Source: CAD feature listing. Evaluate the final solid. Frame: model axes, mm. A direction names the side the tool comes from. Round coordinates to 2 decimals unless told otherwise and drop trailing zeros. Order: outer loops, then holes, each group sorted by start corner. A loop starts at its lowest first (then second) coordinate and runs counter-clockwise, first axis right, second up. Notation, with made-up numbers: M 45,45 L 66,45 A4 cw 66,52 Z; hole C 76,72.5 d3. An arc over 180 degrees is marked long. Answer as CSV lines item,"result". Start each with the question number.
Item 1: Section query A-A on z = 0. Return the cut outline in (x, y), plus the area to 3 significant figures.
Item 2: First-contact query: P1, Ø8, axis at x = 7.5, z = -4, coming from the -Y side; P2, Ø2.5, axis at x = 6.36, z = -6.36, coming from the -Y side; P3, Ø10, axis at y = 29.5, z = -3, coming from the -X side. Flat tips, straight axial feed; report the tip coordinate or a pass-through.
Item 3: Section query C-C on z = -9.5. Return the cut outline in (x, y).
Item 4: Line query: line 1 (Y direction, x = 5.25, z = -6.5); line 2 (Z direction, x = 2, y = 15); line 3 (Y direction, x = 6, z = -6.5). Output: solid intervals per line, ascending. Write a range as [from, to].
Item 5: Section query D-D on z = -4.25. Return the cut outline in (x, y).
Item 6: Section query B-B on y = 23. Return the cut outline in (x, z).
Item 7: Set-up query: faces 4 (the face through (-6, -1, 0)), 5 (the face through (0, -1, -7)), 6 (the face through (5.57, 1.48, -6.97)), 7 (the face through (2.341, 39.544, -10.543)). Return all of +Z, -Z, +X, -X, +Y, -Y with unobstructed straight access to the full face (end or side cutting, diameter ignored); none if empty.
Item 8: Pull-direction query (X, two-part tool) for faces 1 (the face through (-6, 3, -6)), 2 (the face through (0, -1, 7)), 3 (the face through (6, -1, 0)); classes: +X half, -X half, draft (parallel to the pull), parting line (faces both ways), or undercut.
from build123d import *

# Parameters (mm, degrees)
F0_R      = 11
F1_DEPTH  = 25
F2_R      = 10.8
F3_DEPTH  = 29.5
F5_DEPTH  = 2
F6_R      = 2
F7_DEPTH  = 14
F9_DEPTH  = 8
F10_SIZE  = 0.49999
F11_R     = 1
F12_DEPTH = 3


# Not quite as in the source:
# - a fillet or chamfer is up to 0.001 mm smaller than in the source, because OpenCascade refuses the exact size


with BuildPart() as f1:
    # F0 (on Front) → F1 (new body)
    with BuildSketch(Plane.XZ):
        Circle(F0_R)
    extrude(amount=-F1_DEPTH)

    # F2 (on face) → F3 (join)
    with BuildSketch(Plane(origin=(0, 25, 0), x_dir=(-1, 0, 0), z_dir=(0, 1, 0))):
        Circle(F2_R)
    extrude(amount=F3_DEPTH)

    # F4 (on face) → F5 (join)
    with BuildSketch(Plane.XZ):
        with BuildLine():
            Line((6, -3.6055512755), (6, 3.6055512755))
            ThreePointArc((6, 3.6055512755), (0, 7), (-6, 3.6055512755))
            Line((-6, 3.6055512755), (-6, -3.6055512755))
            ThreePointArc((-6, -3.6055512755), (0, -7), (6, -3.6055512755))
        make_face()
    extrude(amount=F5_DEPTH)

    # F6 (on face) → F7 (join)
    with BuildSketch(Plane.XZ.offset(2)):
        Circle(F6_R)
    extrude(amount=F7_DEPTH)

    # F8 (on face) → F9 (cut)
    with BuildSketch(Plane.XZ.offset(16)):
        with BuildLine():
            ThreePointArc((-1.3228756555, -1.5), (0, -2), (1.3228756555, -1.5))
            Line((1.3228756555, -1.5), (-1.3228756555, -1.5))
        make_face()
    extrude(amount=-F9_DEPTH, mode=Mode.SUBTRACT)

    # F10 (size 0.5 in the source; OpenCascade refuses exactly that, so slightly less here)
    f10_edges = [f1.edges().sort_by_distance(p)[0] for p in [
        (0, -8, -1.5),
    ]]
    chamfer(f10_edges, length=F10_SIZE)

    # F11 (on face) → F12 (cut)
    with BuildSketch(Plane.XZ):
        with Locations((6.3639610307, -6.3639610307)):
            Circle(F11_R)
        with Locations((-6.3639610307, -6.3639610307)):
            Circle(F11_R)
        with Locations((-6.3639610307, 6.3639610307)):
            Circle(F11_R)
        with Locations((6.3639610307, 6.3639610307)):
            Circle(F11_R)
    extrude(amount=-F12_DEPTH, mode=Mode.SUBTRACT)


solid = f1.part
Results:
1,outline,"M -11,0 L -6,0 L -6,-2 L -2,-2 L -2,-16 L 2,-16 L 2,-2 L 6,-2 L 6,0 L 11,0 L 11,25 L 10.8,25 L 10.8,54.5 L -10.8,54.5 L -10.8,25 L -11,25 Z"
1,area,"1,270 mm^2"
2,P1,"y = -2"
2,P2,"y = 0"
2,P3,"x = -10.97"
3,outline,"M -5.55,0 L 5.55,0 L 5.55,25 L 5.14,25 L 5.14,54.5 L -5.14,54.5 L -5.14,25 L -5.55,25 Z"
4,line 1,"[0, 54.5]"
4,line 2,"[-10.82, 10.82]"
4,line 3,"[3, 54.5]"
5,outline,"M -10.15,0 L -5.56,0 L -5.56,-2 L 5.56,-2 L 5.56,0 L 10.15,0 L 10.15,25 L 9.93,25 L 9.93,54.5 L -9.93,54.5 L -9.93,25 L -10.15,25 Z"
6,outline,"C 0,0 d22"
7,face 4,"+Z, -Z, -X, -Y"
7,face 5,"-Z, -Y"
7,face 6,"-Y"
7,face 7,"+Y"
8,face 1,"undercut"
8,face 2,"parting line"
8,face 3,"+X half"
